Read the model definition and answer for the solid it produces. Units are mm, in the model's axes. A direction names the side the tool comes from. Round coordinates to 2 decimals unless told otherwise and drop trailing zeros. Order: outer loops, then holes, each group sorted by start corner. A loop starts at its lowest first (then second) coordinate and runs counter-clockwise, first axis right, second up.
from build123d import *

# Parameters (mm, degrees)
SKETCH1_W           = 100
SKETCH1_H           = 45
BOSS_EXTRUDE1_DEPTH = 8
SKETCH2_R           = 1.75
CUT_EXTRUDE1_DEPTH  = 8
SKETCH3_R           = 3.5
CUT_EXTRUDE2_DEPTH  = 3.5
SKETCH4_W           = 30
SKETCH4_H           = 12
BOSS_EXTRUDE2_DEPTH = 55
SKETCH7_W           = 15
SKETCH7_H           = 45
CUT_EXTRUDE4_DEPTH  = 8
SKETCH9_R           = 1.75
CUT_EXTRUDE6_DEPTH  = 12
FILLET1_R           = 10
FILLET2_R           = 10
SKETCH10_R          = 3.5
CUT_EXTRUDE7_DEPTH  = 4


with BuildPart() as part:
    # Sketch1 → Boss-Extrude1 (new body)
    with BuildSketch(Plane(origin=(0, 0, 0), x_dir=(1, 0, 0), z_dir=(0, 1, 0))):
        Rectangle(SKETCH1_W, SKETCH1_H)
    extrude(amount=BOSS_EXTRUDE1_DEPTH)

    # Sketch2 → Cut-Extrude1 (cut)
    with BuildSketch(Plane(origin=(0, 8, 0), x_dir=(1, 0, 0), z_dir=(0, 1, 0))):
        with Locations(Location((20, 15, 0), (0, 0, 270))):
            Circle(SKETCH2_R)
        with Locations(Location((20, -15, 0), (0, 0, 270))):
            Circle(SKETCH2_R)
        with Locations(Location((0, 15, 0), (0, 0, 270))):
            Circle(SKETCH2_R)
        with Locations(Location((0, -15, 0), (0, 0, 270))):
            Circle(SKETCH2_R)
        with Locations(Location((-20, 15, 0), (0, 0, 270))):
            Circle(SKETCH2_R)
        with Locations(Location((-20, -15, 0), (0, 0, 270))):
            Circle(SKETCH2_R)
        with Locations(Location((-40, 15, 0), (0, 0, 270))):
            Circle(SKETCH2_R)
        with Locations(Location((-40, -15, 0), (0, 0, 270))):
            Circle(SKETCH2_R)
    extrude(amount=-CUT_EXTRUDE1_DEPTH, mode=Mode.SUBTRACT)

    # Sketch3 → Cut-Extrude2 (cut)
    with BuildSketch(Plane(origin=(0, 8, 0), x_dir=(1, 0, 0), z_dir=(0, 1, 0))):
        with Locations(Location((-40, 15, 0), (0, 0, 270))):
            Circle(SKETCH3_R)
        with Locations(Location((-20, 15, 0), (0, 0, 270))):
            Circle(SKETCH3_R)
        with Locations(Location((0, 15, 0), (0, 0, 270))):
            Circle(SKETCH3_R)
        with Locations(Location((20, 15, 0), (0, 0, 270))):
            Circle(SKETCH3_R)
        with Locations(Location((-40, -15, 0), (0, 0, 270))):
            Circle(SKETCH3_R)
        with Locations(Location((-20, -15, 0), (0, 0, 270))):
            Circle(SKETCH3_R)
        with Locations(Location((0, -15, 0), (0, 0, 270))):
            Circle(SKETCH3_R)
        with Locations(Location((20, -15, 0), (0, 0, 270))):
            Circle(SKETCH3_R)
    extrude(amount=-CUT_EXTRUDE2_DEPTH, mode=Mode.SUBTRACT)

    # Sketch4 → Boss-Extrude2 (add)
    with BuildSketch(Plane(origin=(0, 8, 0), x_dir=(1, 0, 0), z_dir=(0, 1, 0))):
        with Locations((14, 0)):
            Rectangle(SKETCH4_W, SKETCH4_H)
    extrude(amount=BOSS_EXTRUDE2_DEPTH)

    # Sketch7 → Cut-Extrude4 (cut)
    with BuildSketch(Plane(origin=(0, 8, 0), x_dir=(1, 0, 0), z_dir=(0, 1, 0))):
        with Locations((42.5, 0)):
            Rectangle(SKETCH7_W, SKETCH7_H)
    extrude(amount=-CUT_EXTRUDE4_DEPTH, mode=Mode.SUBTRACT)

    # Sketch9 → Cut-Extrude6 (cut)
    with BuildSketch(Plane(origin=(0, 0, -6), x_dir=(-1, 0, 0), z_dir=(0, 0, -1))):
        with Locations((-14, 56)):
            Circle(SKETCH9_R)
        with Locations((-14, 36)):
            Circle(SKETCH9_R)
    extrude(amount=-CUT_EXTRUDE6_DEPTH, mode=Mode.SUBTRACT)

    # Fillet1
    fillet1_edges = [part.edges().sort_by_distance(p)[0] for p in [
        (29, 63, 0),
    ]]
    fillet(fillet1_edges, radius=FILLET1_R)

    # Fillet2
    fillet2_edges = [part.edges().sort_by_distance(p)[0] for p in [
        (-1, 63, 0),
    ]]
    fillet(fillet2_edges, radius=FILLET2_R)

    # Sketch10 → Cut-Extrude7 (cut)
    with BuildSketch(Plane.XY.offset(6)):
        with Locations((14, 36)):
            Circle(SKETCH10_R)
        with Locations((14, 56)):
            Circle(SKETCH10_R)
    extrude(amount=-CUT_EXTRUDE7_DEPTH, mode=Mode.SUBTRACT)


solid = part.part
Q1. A cutting plane is placed at A-A, the plane x = -20. Give the vertices of the cut face in (y, z).
Outcome:
outline: (0, -22.5) - (8, -22.5) - (8, -18.5) - (4.5, -18.5) - (4.5, -16.75) - (0, -16.75) - close; (0, -13.25) - (4.5, -13.25) - (4.5, -11.5) - (8, -11.5) - (8, 11.5) - (4.5, 11.5) - (4.5, 13.25) - (0, 13.25) - close; (0, 16.75) - (4.5, 16.75) - (4.5, 18.5) - (8, 18.5) - (8, 22.5) - (0, 22.5) - close
Q2. A cutting plane is placed at C-C, the plane y = 56. Give the vertices of the cut face in (x, z), plus the area to 3 significant figures.
Outcome:
outline: (-0.54, -6) - (12.25, -6) - (12.25, 2) - (10.5, 2) - (10.5, 6) - (-0.54, 6) - close; (15.75, -6) - (28.54, -6) - (28.54, 6) - (17.5, 6) - (17.5, 2) - (15.75, 2) - close
area: 293 mm2
Q3. For a pull along Z with two mould halves and no side action, classify faces 1 (the face through (17.34, 57.05, 4.03)), 2 (the face through (-8, 4, 22.5)), 3 (the face through (-41, 4.5, -17)) as released by +Z, released by -Z, zero draft, split by the parting line, or undercut.
Outcome:
face 1: zero draft
face 2: released by +Z
face 3: undercut
Q4. A cutting plane is placed at B-B, the plane z = 4. Give the vertices of the cut face in (x, y), plus the area to 3 significant figures.
Outcome:
outline: (-50, 0) - (35, 0) - (35, 8) - (29, 8) - (29, 53) arc R10 ccw to (19, 63) - (9, 63) arc R10 ccw to (-1, 53) - (-1, 8) - (-50, 8) - close; hole circle Ø7 at (14, 36); hole circle Ø7 at (14, 56)
area: 2,210 mm2
Q5. Flat-ended cylindrical pins translate along their axes: pin 1 (3 mm diameter, centred on x = -40, z = -15, fed in from -Y); pin 2 (13 mm diameter, centred on y = 31.5, z = -2.5, fed in from +X); pin 3 (4 mm diameter, centred on x = 14, y = 36, fed in from +Z); pin 4 (1.5 mm diameter, centred on x = 6.5, y = 14, fed in from +Z). Find the tip coordinate at first contact, or state that the pin passes through.
Outcome:
pin 1: passes through
pin 2: stops at x = 29
pin 3: stops at z = 2
pin 4: stops at z = 6
Q6. For faces 4 (the face through (29, 30, 0)), 5 (the face through (10, 35, 6)), 6 (the face through (-50, 4, 0)), 7 (the face through (-36.53, 6.27, -15.46)), determine the directions among +Z, -Z, +X, -X, +Y, -Y from which every point of the face is accessible in a straight line to the end or side of a thin tool.
Outcome:
face 4: +Z, -Z, +X, +Y
face 5: +Z, +X, -X, +Y
face 6: +Z, -Z, -X, +Y, -Y
face 7: +Y
Q7. Straight lines are drawn through the part: probe 1 along X at (y, z) = (3, -15); probe 2 along Y at (x, z) = (14, 3); probe 3 along Y at (x, z) = (14, -1). For each, find the intervals that lie inside material, in ascending order.
Outcome:
probe 1: x = -50 to -41.75, -38.25 to -21.75, -18.25 to -1.75, 1.75 to 18.25, 21.75 to 35
probe 2: y = 0 to 32.5, 39.5 to 52.5, 59.5 to 63
probe 3: y = 0 to 34.25, 37.75 to 54.25, 57.75 to 63
Q8. A cutting plane is placed at D-D, the plane z = -15. Give the number of separate pieces and of enclosed holes in the cut face, plus the area to 3 significant figures.
Outcome:
separate pieces: 5
enclosed holes: 0
area: 519 mm2
